The drawing under review shows one solid part. Ordinate dimensions are in mm from its lowest x, y, z. Give positions to 0.01 mm unless a question says otherwise; leave off trailing zeros. Loops run counter-clockwise (first coordinate to the right, second up) from the corner with the lowest first, then second, coordinate; pieces in that order, holes last. Notation, with made-up numbers: M -1.75,59.25 L 2.25,59.25 A17 ccw 2.25,85.25 Z; hole C -15,-5 d10. An arc over 180 degrees is marked long. One line per item, written item: value. Start each with the question number.
Q1. To check wall thickness, follow line 1 along Z through (x, y) = (8.5, 17.5); line 2 along Y through (x, z) = (16.25, 12); line 3 along Y through (x, z) = (6, 14). State the ranges of each line that lie inside material, in increasing order. Write a range as from..to.
Q2. We need section C-C on x = 1.5. Write out the cut boundary in (y, z).
Q3. For pin 1 (6 mm diameter, centred on x = 4.5, z = 6, fed in from +Y); pin 2 (12 mm diameter, centred on x = 17.5, z = 27.5, fed in from -Y); pin 3 (2 mm diameter, centred on x = 9.5, z = 19.5, fed in from -Y), all flat-tipped, find the tip position at first contact; note any pin that passes through.
Q4. We need section A-A on z = 17.5. Write out the cut boundary in (x, y), plus the area to 3 significant figures.
Q5. Mouldability with a two-part tool opening along Z and no side actions: class the marked faces 1 and 2 as released by +Z, released by -Z, zero draft, split by the parting line, or undercut.
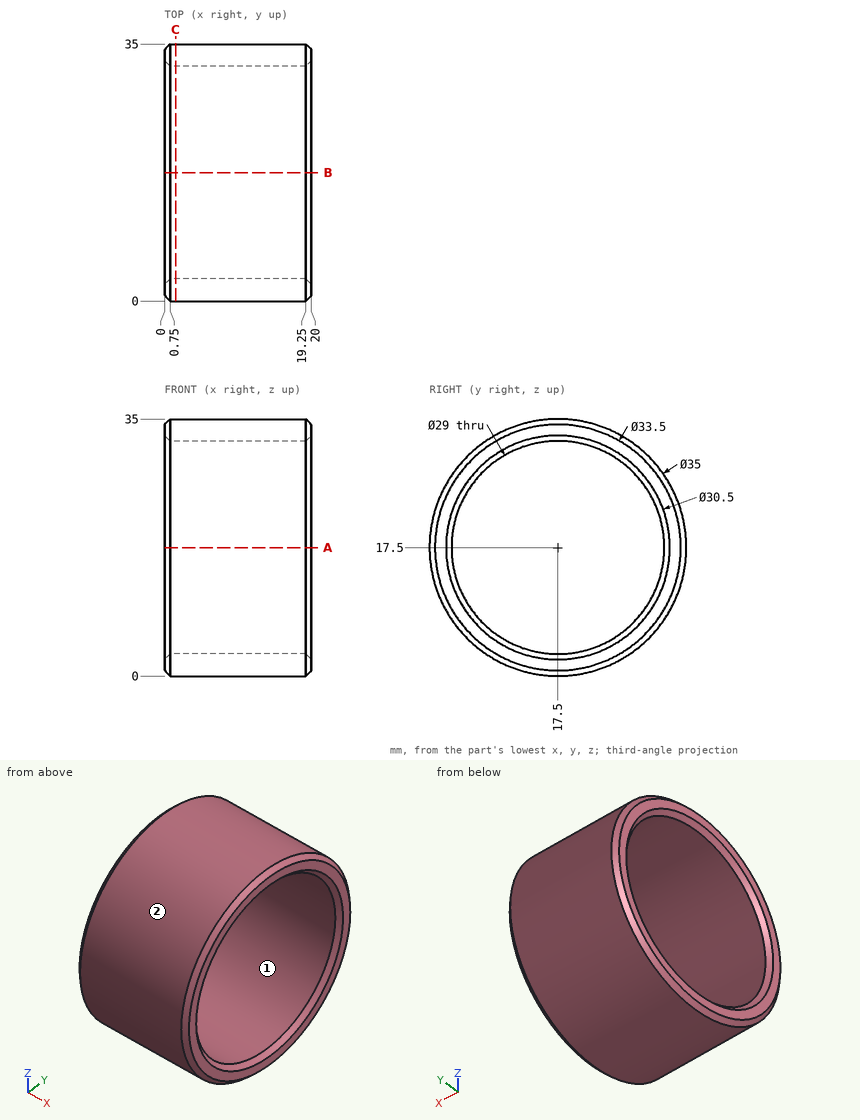
Solved:
1. line 1: 0..3, 32..35
1. line 2: 0.89..4.08, 30.92..34.11
1. line 3: 0.35..3.43, 31.57..34.65
2. outline: C 17.5,17.5 d35; hole C 17.5,17.5 d29
3. pin 1: y = 32.8
3. pin 2: y = 0.46
3. pin 3: y = 0.03
4. outline: M 0,0.75 L 0.75,0 L 19.25,0 L 20,0.75 L 20,2.25 L 19.25,3 L 0.75,3 L 0,2.25 Z; M 0,32.75 L 0.75,32 L 19.25,32 L 20,32.75 L 20,34.25 L 19.25,35 L 0.75,35 L 0,34.25 Z
4. area: 118 mm2
5. face 1: undercut
5. face 2: split by the parting line
